For this review, use the dimensioned drawing (mm, ordinates from the lowest corner) and the shaded views. A direction names the side the tool comes from. Round coordinates to 2 decimals unless told otherwise and drop trailing zeros. Loops run counter-clockwise (first coordinate to the right, second up) from the corner with the lowest first, then second, coordinate; pieces in that order, holes last. Notation, with made-up numbers: (-21, -12.5) -> (-7, -12.5) arc R14 ccw to (-7, -3.5) -> close; hole circle Ø10 at (-6, 0.25). An arc over 180 degrees is marked (long way). Answer as CSV lines item,"result". Start each with the question number.
(1) Take a section at B-B, the plane z = 6. Write out the cut boundary in (x, y).
(2) Machinability: for the marked faces 1, 2 and 3, which of the approach directions +Z, -Z, +X, -X, +Y, -Y give a long, thin tool a straight path to every point of the face, cutting with its end or side? Answer none if there is none.
(3) Take a section at D-D, the plane y = 18.5. Write out the cut boundary in (x, z), and give its area (3 significant figures).
(4) Take a section at A-A, the plane x = 8.75. Write out the cut boundary in (y, z).
(5) Take a section at C-C, the plane x = 13.5. Write out the cut boundary in (y, z) (1 decimal).
(6) To check wall thickness, follow line 1 (Z direction, x = 10.5, y = 4.75); line 2 (Y direction, x = 11.25, z = 16.5); line 3 (Z direction, x = 4, y = 22.6) (1 decimal). State the ranges of each line that lie inside material, in increasing order. Write a range as from..to.
(7) For P1, Ø9, axis at x = 8.5, y = 14.5, coming from the -Z side; P2, Ø1.5, axis at x = 12.5, y = 18, coming from the +Z side; P3, Ø2, axis at x = 4, z = 8, coming from the +Y side, all flat-tipped, find the tip position at first contact; note any pin that passes through.
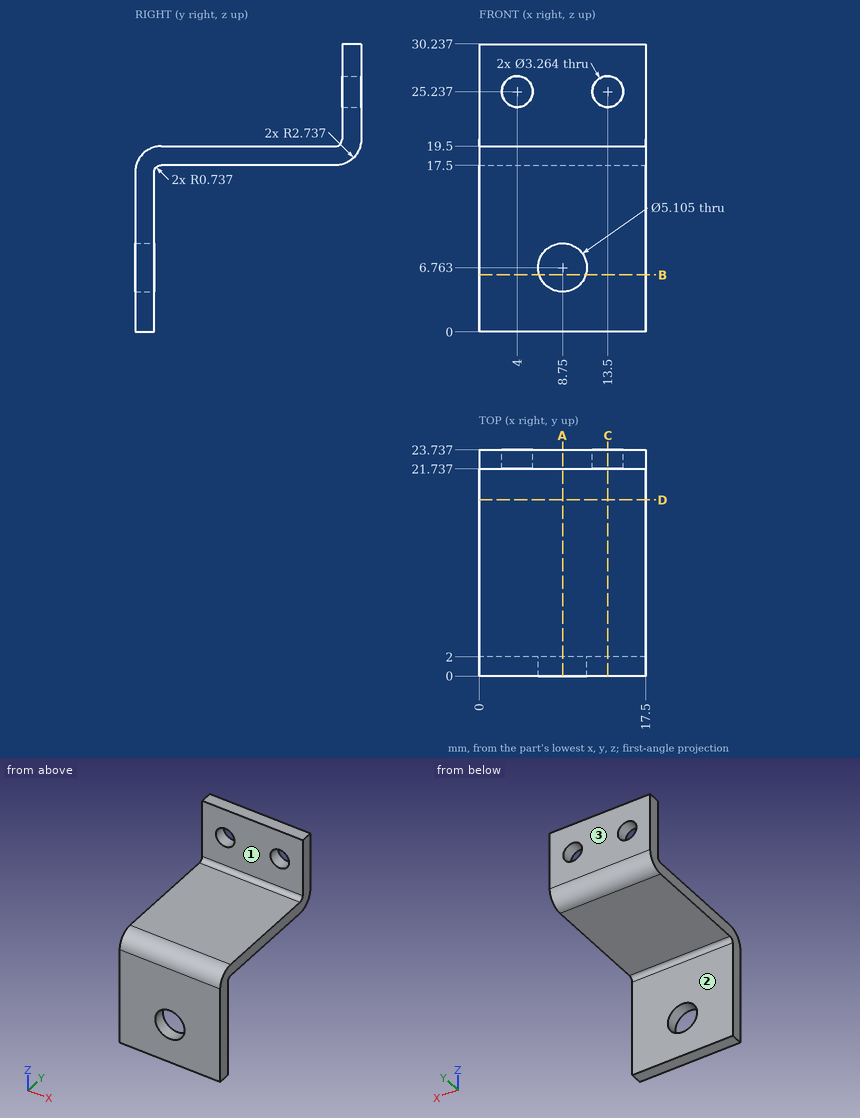
The answers:
1,outline,"(0, 0) -> (6.31, 0) -> (6.31, 2) -> (0, 2) -> close; (11.19, 0) -> (17.5, 0) -> (17.5, 2) -> (11.19, 2) -> close"
2,face 1,"+Z, +X, -X, -Y"
2,face 2,"-Z, +X, -X, +Y"
2,face 3,"+Z, -Z, +X, -X, +Y"
3,outline,"(0, 17.5) -> (17.5, 17.5) -> (17.5, 19.5) -> (0, 19.5) -> close"
3,area,"35.0 mm²"
4,outline,"(0, 0) -> (2, 0) -> (2, 4.21) -> (0, 4.21) -> close; (0, 9.32) -> (2, 9.32) -> (2, 16.76) arc R0.74 cw to (2.74, 17.5) -> (21, 17.5) arc R2.74 ccw to (23.74, 20.24) -> (23.74, 30.24) -> (21.74, 30.24) -> (21.74, 20.24) arc R0.74 cw to (21, 19.5) -> (2.74, 19.5) arc R2.74 ccw to (0, 16.76) -> close"
5,outline,"(0, 0) -> (2, 0) -> (2, 16.8) arc R0.7 cw to (2.7, 17.5) -> (21, 17.5) arc R2.7 ccw to (23.7, 20.2) -> (23.7, 23.6) -> (21.7, 23.6) -> (21.7, 20.2) arc R0.7 cw to (21, 19.5) -> (2.7, 19.5) arc R2.7 ccw to (0, 16.8) -> close; (21.7, 26.9) -> (23.7, 26.9) -> (23.7, 30.2) -> (21.7, 30.2) -> close"
6,line 1,"17.5..19.5"
6,line 2,"0..2"
6,line 3,"18..23.6, 26.9..30.2"
7,P1,"z = 17.5"
7,P2,"z = 19.5"
7,P3,"y = 2"
